```python
from build123d import *

# Parameters (mm, degrees)
SKETCH_1_R      = 1.5
SKETCH_1_R_2    = 2
EXTRUDE_1_DEPTH = 3
FILLET_1_R      = 3


with BuildPart() as part:
    # 草图1 → 凸台-拉伸1 (new body)
    with BuildSketch(Plane(origin=(0, 0, 0), x_dir=(1, 0, 0), z_dir=(0, 1, 0))):
        with BuildLine():
            Line((51.058349832, 23), (-41.5, 23))
            Line((-41.5, 23), (-41.5, -23))
            Line((-41.5, -23), (-3.963622721, -46.367078995))
            ThreePointArc((-3.963622721, -46.367078995), (0.137420172, -47.498740941), (4.194246234, -46.217579797))
            Line((4.194246234, -46.217579797), (46.024182835, -18))
            Line((46.024182835, -18), (51.058349832, 23))
        make_face()
        with Locations(Location((-36.5, 18, 0), (0, 0, 270))):
            Circle(SKETCH_1_R, mode=Mode.SUBTRACT)
        with Locations(Location((36.5, 18, 0), (0, 0, 270))):
            Circle(SKETCH_1_R, mode=Mode.SUBTRACT)
        with Locations(Location((36.5, -18, 0), (0, 0, 270))):
            Circle(SKETCH_1_R, mode=Mode.SUBTRACT)
        with Locations(Location((-36.5, -18, 0), (0, 0, 270))):
            Circle(SKETCH_1_R, mode=Mode.SUBTRACT)
        with Locations(Location((0, -40, 0), (0, 0, 270))):
            Circle(SKETCH_1_R_2, mode=Mode.SUBTRACT)
        with Locations(Location((46.160921266, 7.730172301, 0), (0, 0, 270))):
            Circle(SKETCH_1_R, mode=Mode.SUBTRACT)
        with Locations(Location((47.3796147, 17.655633817, 0), (0, 0, 270))):
            Circle(SKETCH_1_R, mode=Mode.SUBTRACT)
        Polygon((-29.717158085, 18), (29.717158085, 18), (0, 3.344963136), align=None, mode=Mode.SUBTRACT)
        Polygon((-36.5, 14.655036864), (-36.5, -14.655036864), (-6.782841915, 0), align=None, mode=Mode.SUBTRACT)
        Polygon((29.717158085, -18), (0, -3.344963136), (-29.717158085, -18), align=None, mode=Mode.SUBTRACT)
        Polygon((36.5, -14.655036864), (6.782841915, 0), (36.5, 14.655036864), align=None, mode=Mode.SUBTRACT)
        with BuildLine():
            Line((-32.038958261, -23), (29.671328196, -23))
            Line((29.671328196, -23), (5.919801281, -39.022271619))
            ThreePointArc((5.919801281, -39.022271619), (-0.109936138, -34.001007247), (-5.951649691, -39.239825052))
            Line((-5.951649691, -39.239825052), (-32.038958261, -23))
        make_face(mode=Mode.SUBTRACT)
    extrude(amount=EXTRUDE_1_DEPTH)

    # 圆角1
    fillet_1_edges = [part.edges().sort_by_distance(p)[0] for p in [
        (-41.5, 1.5, 23),
        (-41.5, 1.5, -23),
        (51.058349832, 1.5, -23),
        (46.024182835, 1.5, 18),
        (-32.038958261, 1.5, 23),
        (-5.951649691, 1.5, 39.239825052),
        (5.919801281, 1.5, 39.022271619),
        (29.671328196, 1.5, 23),
        (-29.717158085, 1.5, -18),
        (0, 1.5, -3.344963136),
        (29.717158085, 1.5, -18),
        (-6.782841915, 1.5, 0),
        (-36.5, 1.5, -14.655036864),
        (-36.5, 1.5, 14.655036864),
        (-29.717158085, 1.5, 18),
        (29.717158085, 1.5, 18),
        (0, 1.5, 3.344963136),
        (36.5, 1.5, 14.655036864),
        (36.5, 1.5, -14.655036864),
        (6.782841915, 1.5, 0),
    ]]
    fillet(fillet_1_edges, radius=FILLET_1_R)


solid = part.part
```
Design review of the part built by this model. Coordinates are the model's own, in mm. A direction names the side the tool comes from. Coordinates: 2 decimals unless noted, no trailing zeros. Write each loop counter-clockwise with the first axis right and the second up, starting at its lowest first coordinate (ties: lowest second). Pieces come first, ordered by that corner, then holes.
1) Mouldability with a two-part tool opening along Z and no side actions: class faces 3 (the flat face through (5, 1, -23)), 4 (the cylindrical face through (0.1, 1.5, 47.5)), 5 (the cylindrical face through (10.566, 1.521, -0.047)) as +Z half, -Z half, draft (parallel to the pull), parting line (faces both ways), or undercut.
2) Add section B-B (z = 40). Write out the cut boundary in (x, y).
3) Machinability: for faces 1 (the flat face through (4, 3, 4)), 2 (the cylindrical face through (-19.785, 1.521, -15.626)), which of the approach directions +Z, -Z, +X, -X, +Y, -Y give a long, thin tool a straight path to every point of the face, cutting with its end or side? Answer none if there is none.
4) Add section A-A (x = 0). Write out the cut boundary in (y, z), plus the area to 3 significant figures.
5) Add section C-C (z = -14). Write out the cut boundary in (x, y), plus the area to 3 significant figures.
6) To check wall thickness, follow L1, parallel to Z at x = -14, y = 2.85; L2, parallel to Z at x = -5, y = 2.3; L3, parallel to X at y = 0.85, z = -11. State the ranges of each line that lie inside material, in increasing order.
7) Add section D-D (y = 1.95). State how many separate pieces and enclosed holes the cut face has, plus the area to 3 significant figures.
Check result:
1. face 3: -Z half
1. face 4: +Z half
1. face 5: undercut
2. outline: (-14.19, 0) - (-2, 0) - (-2, 3) - (-14.19, 3) - close; (2, 0) - (13.41, 0) - (13.41, 3) - (2, 3) - close
3. face 1: +Z, -Z, +X, -X, +Y
3. face 2: +Y, -Y
4. outline: (0, -23) - (3, -23) - (3, -18) - (0, -18) - close; (0, -3.69) - (3, -3.69) - (3, 3.69) - (0, 3.69) - close; (0, 18) - (3, 18) - (3, 23) - (0, 23) - close; (0, 34) - (3, 34) - (3, 38) - (0, 38) - close; (0, 42) - (3, 42) - (3, 47.5) - (0, 47.5) - close
4. area: 80.6 mm2
5. outline: (-41.5, 0) - (-19.68, 0) - (-19.68, 3) - (-41.5, 3) - close; (19.68, 0) - (49.95, 0) - (49.95, 3) - (19.68, 3) - close
5. area: 156 mm2
6. L1: z = -23 to -18, -10.25 to -3.56, 3.56 to 10.25, 18 to 23, 34.23 to 40.12
6. L2: z = -23 to -18, -5.81 to 5.81, 18 to 23, 36.67 to 45.72
6. L3: x = -41.5 to -36.26, -29.09 to -15.52, 15.52 to 29.09, 36.26 to 49.58
7. separate pieces: 1
7. enclosed holes: 12
7. area: 2,980 mm2
